```python
from build123d import *

# Parameters (mm, degrees)
F0_W     = 1828.8
F0_H     = 304.8
F1_DEPTH = 355.6
F2_T     = -12.7
F4_DEPTH = 342.9
F5_R     = 25.4
F6_DEPTH = 190.5


with BuildPart() as f1:
    # F0 (on Front) → F1 (new body)
    with BuildSketch(Plane.XZ):
        Rectangle(F0_W, F0_H)
    extrude(amount=F1_DEPTH)

    # F2
    f2_openings = [f1.faces().sort_by_distance(p)[0] for p in [
        (0, -355.6, 0),
    ]]
    offset(amount=F2_T, openings=f2_openings)

    # F3 (on face) → F4 (join)
    with BuildSketch(Plane.XZ.offset(12.7)):
        Polygon((12.7, 12.7), (12.7, 139.7), (-12.7, 139.7), (-12.7, 12.7), (-901.7, 12.7), (-901.7, -12.7), (-12.7, -12.7), (-12.7, -139.7), (12.7, -139.7), (12.7, -12.7), (901.7, -12.7), (901.7, 12.7), align=None)
    extrude(amount=F4_DEPTH)

    # F5 (on face) → F6 (cut)
    with BuildSketch(Plane.XY.offset(152.4)):
        with Locations((-762, -177.8)):
            Circle(F5_R)
        with Locations((762, -177.8)):
            Circle(F5_R)
    extrude(amount=-F6_DEPTH, mode=Mode.SUBTRACT)


solid = f1.part
```
The listing builds one solid part. Answer for the finished solid, in the listing's coordinates (mm). A direction names the side the tool comes from. Coordinates: 2 decimals unless noted, no trailing zeros. Loops run counter-clockwise (first coordinate to the right, second up) from the corner with the lowest first, then second, coordinate; pieces in that order, holes last. Notation, with made-up numbers: (86.5, -15) -> (120.5, -15) arc R6 ccw to (120.5, -6) -> close; hole circle Ø4 at (-14, -38.5). An arc over 180 degrees is marked (long way). Use one line per item in the form item = value. Start each with the question number.
Item 1: A tool of negligible diameter and unlimited length cuts with its end or side. For faces 1 (the face through (-737.773, -170.171, 0.178)), 2 (the face through (-13, 0, 2)), 3 (the face through (901.7, -182, 75)), from which of +Z, -Z, +X, -X, +Y, -Y can it reach the whole face along a straight path? Write none if from no direction.
Item 2: Consider L1, parallel to X at y = -315, z = 95; L2, parallel to Z at x = 204, y = -112; L3, parallel to X at y = -177, z = -6. Determine where each line is inside the solid, lowest interval first. Write a range as [from, to].
Item 3: The part is cut by section D-D on z = -104. Determine the outline of the cut face in (x, y).
Item 4: The part is cut by section A-A on x = 762. Determine the outline of the cut face in (y, z).
Item 5: The mould has two halves that part along X. Classify faces 4 (the face through (-914.4, -175, -2)), 5 (the face through (786.227, -170.171, 0.178)), 6 (the face through (-13, -175, -152.4)): released by +X, released by -X, zero draft, split by the parting line, or undercut.
Item 6: A flat-ended cylindrical pin translates along its axis: pin 1 Ø12 at (x, z) = (217, 105) entering from -Y. Find the tip coordinate at first contact, or state that the pin passes through.
Item 7: The part is cut by section B-B on y = -315. Determine the outline of the cut face in (x, z), then the cut area to 3 significant figures.
Item 8: The part is cut by section C-C on x = -103. Determine the outline of the cut face in (y, z).
Answer key:
q1.face_1 = +Z
q1.face_2 = +Z, -Z, +X, -X, +Y
q1.face_3 = -Y
q2.L1 = [-914.4, -901.7], [-12.7, 12.7], [901.7, 914.4]
q2.L2 = [-152.4, -139.7], [-12.7, 12.7], [139.7, 152.4]
q2.L3 = [-914.4, -787.39], [-736.61, 736.61], [787.39, 914.4]
q3.outline = (-914.4, -355.6) -> (-901.7, -355.6) -> (-901.7, -12.7) -> (-12.7, -12.7) -> (-12.7, -355.6) -> (12.7, -355.6) -> (12.7, -12.7) -> (901.7, -12.7) -> (901.7, -355.6) -> (914.4, -355.6) -> (914.4, 0) -> (-914.4, 0) -> close
q4.outline = (-355.6, -152.4) -> (0, -152.4) -> (0, 152.4) -> (-152.4, 152.4) -> (-152.4, 139.7) -> (-12.7, 139.7) -> (-12.7, 12.7) -> (-152.4, 12.7) -> (-152.4, -12.7) -> (-12.7, -12.7) -> (-12.7, -139.7) -> (-355.6, -139.7) -> close; (-355.6, -12.7) -> (-203.2, -12.7) -> (-203.2, 12.7) -> (-355.6, 12.7) -> close; (-355.6, 139.7) -> (-203.2, 139.7) -> (-203.2, 152.4) -> (-355.6, 152.4) -> close
q5.face_4 = released by -X
q5.face_5 = undercut
q5.face_6 = zero draft
q6.pin_1 = -12.7
q7.outline = (-914.4, -152.4) -> (914.4, -152.4) -> (914.4, 152.4) -> (-914.4, 152.4) -> close; hole (-901.7, -139.7) -> (-12.7, -139.7) -> (-12.7, -12.7) -> (-901.7, -12.7) -> close; hole (-901.7, 12.7) -> (-12.7, 12.7) -> (-12.7, 139.7) -> (-901.7, 139.7) -> close; hole (12.7, -139.7) -> (901.7, -139.7) -> (901.7, -12.7) -> (12.7, -12.7) -> close; hole (12.7, 12.7) -> (901.7, 12.7) -> (901.7, 139.7) -> (12.7, 139.7) -> close
q7.area = 106,000 mm2
q8.outline = (-355.6, -152.4) -> (0, -152.4) -> (0, 152.4) -> (-355.6, 152.4) -> (-355.6, 139.7) -> (-12.7, 139.7) -> (-12.7, 12.7) -> (-355.6, 12.7) -> (-355.6, -12.7) -> (-12.7, -12.7) -> (-12.7, -139.7) -> (-355.6, -139.7) -> close
